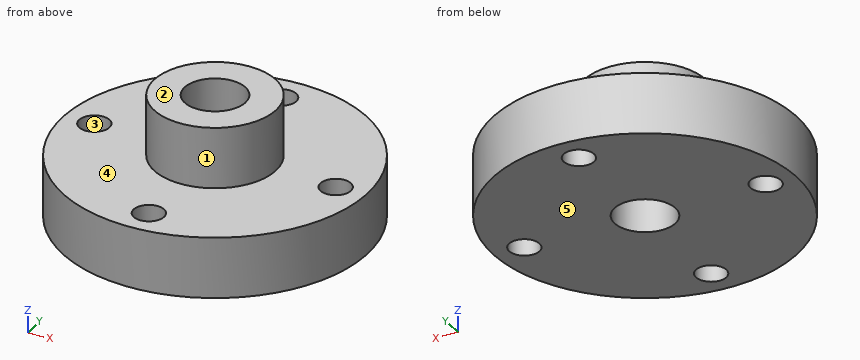
```python
from build123d import *

# Parameters (mm, degrees)
F0_R     = 31.75
F0_R_2   = 12.7
F1_DEPTH = 12.7
F0_R_3   = 6.35
F2_DEPTH = 25.4
F4_D     = 6.35


with BuildPart() as f1:
    # F0 (on Top) → F1 (new body)
    with BuildSketch(Plane.XY):
        Circle(F0_R)
        Circle(F0_R_2, mode=Mode.SUBTRACT)
    extrude(amount=F1_DEPTH)

    # F0 (on Top) → F2 (join)
    with BuildSketch(Plane.XY):
        Circle(F0_R_2)
        Circle(F0_R_3, mode=Mode.SUBTRACT)
    extrude(amount=F2_DEPTH)

    # F4 (through all)
    with Locations(Plane.XY.offset(12.7)):
        with Locations((0, 25.4), (25.4, 0), (0, -25.4), (-25.4, 0)):
            Hole(F4_D / 2)


solid = f1.part
```
Geometry check sheet. Reference: the model listing, model coordinates, mm. Face numbers are marked on the shaded views. A direction names the side the tool comes from. Give positions to 0.01 mm unless a question says otherwise; leave off trailing zeros. Order: outer loops, then holes, each group sorted by start corner. A loop starts at its lowest first (then second) coordinate and runs counter-clockwise, first axis right, second up. Notation, with made-up numbers: (24, 66.5) - (80, 66.5) arc R31 ccw to (80, 92.5) - close; hole circle Ø4 at (-9, 30.25). An arc over 180 degrees is marked (long way). Answer in a Markdown table with one row per item. Add a question column.
Q1. Mould release check, pull along X, two halves, no side actions. Record for the marked faces 1, 2 and 3: pulls with the +X half, pulls with the -X half, needs draft (parallel to the pull), parting line crosses it, or undercut.
Q2. Cross-section at A-A, the plane x = -25.4. Enter the section's corners in (y, z) (3 decimals), then the cut area to 3 significant figures.
Q3. Cross-section at B-B, the plane y = 0. Enter the section's corners in (x, z) (3 decimals).
Q4. Material ranges on probe 1 along Y at (x, z) = (0, 10.5) (3 decimals); probe 2 along X at (y, z) = (-1, 1.5); probe 3 along Z at (x, y) = (8.5, -25), recorded low to high. Write a range as from..to.
Q5. Tool access check on the marked faces 4 and 5. Record the directions out of +Z, -Z, +X, -X, +Y, -Y that give a thin tool (end or side, any length) a straight path to the whole face; none if there is none.
Q6. Gauge pin test, flat ends, axial feed: pin 1 (6 mm diameter, centred on y = -10.5, z = 4, fed in from +X); pin 2 (12 mm diameter, centred on x = 18.5, y = -5, fed in from +Z); pin 3 (4 mm diameter, centred on y = 18, z = 12, fed in from -X). Record the tip position at first contact, or that the pin passes through.
Check values:
| question | item | result |
|---|---|---|
| 1 | face 1 | parting line crosses it |
| 1 | face 2 | needs draft |
| 1 | face 3 | undercut |
| 2 | outline | (-19.05, 0) - (-3.175, 0) - (-3.175, 12.7) - (-19.05, 12.7) - close; (3.175, 0) - (19.05, 0) - (19.05, 12.7) - (3.175, 12.7) - close |
| 2 | area | 403 mm^2 |
| 3 | outline | (-31.75, 0) - (-28.575, 0) - (-28.575, 12.7) - (-31.75, 12.7) - close; (-22.225, 0) - (-6.35, 0) - (-6.35, 25.4) - (-12.7, 25.4) - (-12.7, 12.7) - (-22.225, 12.7) - close; (6.35, 0) - (22.225, 0) - (22.225, 12.7) - (12.7, 12.7) - (12.7, 25.4) - (6.35, 25.4) - close; (28.575, 0) - (31.75, 0) - (31.75, 12.7) - (28.575, 12.7) - close |
| 4 | probe 1 | y = -31.75..-28.575, -22.225..-6.35, 6.35..22.225, 28.575..31.75 |
| 4 | probe 2 | x = -31.73..-28.41, -22.39..-6.27, 6.27..22.39, 28.41..31.73 |
| 4 | probe 3 | z = 0..12.7 |
| 5 | face 4 | +Z |
| 5 | face 5 | -Z, +X, -X, +Y, -Y |
| 6 | pin 1 | stops at x = 30.85 |
| 6 | pin 2 | stops at z = 12.7 |
| 6 | pin 3 | stops at x = -27.42 |
